For this review, take the finished solid that the model builds, in its own axes (mm). A direction names the side the tool comes from. Give positions to 0.01 mm unless a question says otherwise; leave off trailing zeros. Write each loop counter-clockwise with the first axis right and the second up, starting at its lowest first coordinate (ties: lowest second). Pieces come first, ordered by that corner, then holes. Notation, with made-up numbers: (53.25, 32.5) -> (111.25, 32.5) arc R28 cw to (111.25, 56.5) -> close; hole circle Ø5 at (61, 17.5). An arc over 180 degrees is marked (long way). Return JSON: item names as keys, results as strings.
from build123d import *

# Parameters (mm, degrees)
SKETCH1_R           = 2
SKETCH1_R_2         = 1.025
BOSS_EXTRUDE1_DEPTH = 3
SKETCH2_R           = 2
BOSS_EXTRUDE2_DEPTH = 1
SKETCH3_R           = 1.575
BOSS_EXTRUDE3_DEPTH = 27


with BuildPart() as part:
    # Sketch1 → Boss-Extrude1 (new body)
    with BuildSketch(Plane(origin=(0, 0, 0), x_dir=(1, 0, 0), z_dir=(0, 1, 0))):
        Circle(SKETCH1_R)
        Circle(SKETCH1_R_2, mode=Mode.SUBTRACT)
    extrude(amount=BOSS_EXTRUDE1_DEPTH)

    # Sketch2 → Boss-Extrude2 (add)
    with BuildSketch(Plane(origin=(0, 3, 0), x_dir=(1, 0, 0), z_dir=(0, 1, 0))):
        Circle(SKETCH2_R)
    extrude(amount=BOSS_EXTRUDE2_DEPTH)

    # Sketch3 → Boss-Extrude3 (add)
    with BuildSketch(Plane(origin=(0, 4, 0), x_dir=(1, 0, 0), z_dir=(0, 1, 0))):
        Circle(SKETCH3_R)
    extrude(amount=BOSS_EXTRUDE3_DEPTH)


solid = part.part
1. The part is to be moulded in two halves that separate along Z. For faces 3 (the cylindrical face through (-0.133, 1.479, -1.016)), 4 (the flat face through (0, 31, 0)), 5 (the cylindrical face through (-1.25, 17.31, 0.96)), say which applies: +Z half, -Z half, draft (parallel to the pull), parting line (faces both ways), or undercut.
Results found:
{"face 3": "undercut", "face 4": "draft", "face 5": "parting line"}
2. For pin 1 (1.5 mm diameter, centred on x = -1, z = 0.5, fed in from -Y); pin 2 (1 mm diameter, centred on x = 0, z = 0, fed in from -Y), all flat-tipped, find the tip position at first contact; note any pin that passes through.
Results found:
{"pin 1": "stops at y = 0", "pin 2": "stops at y = 3"}
3. Add section C-C, the plane y = 4.5. State the section outline as (x, z) points (3 decimals), plus the area to 3 significant figures.
Results found:
{"outline": "circle Ø3.15 at (0, 0)", "area": "7.79 mm²"}
4. Add section B-B, the plane x = 0. State the section outline as (y, z) points (3 decimals), plus the area to 3 significant figures.
Results found:
{"outline": "(0, -2) -> (4, -2) -> (4, -1.575) -> (31, -1.575) -> (31, 1.575) -> (4, 1.575) -> (4, 2) -> (0, 2) -> (0, 1.025) -> (3, 1.025) -> (3, -1.025) -> (0, -1.025) -> close", "area": "94.9 mm²"}
5. Add section A-A, the plane z = 0. State the section outline as (x, y) points (3 decimals), plus the area to 3 significant figures.
Results found:
{"outline": "(-2, 0) -> (-1.025, 0) -> (-1.025, 3) -> (1.025, 3) -> (1.025, 0) -> (2, 0) -> (2, 4) -> (1.575, 4) -> (1.575, 31) -> (-1.575, 31) -> (-1.575, 4) -> (-2, 4) -> close", "area": "94.9 mm²"}
6. To check wall thickness, follow probe 1 along X at (y, z) = (1.4, 0) (3 decimals); probe 2 along Y at (x, z) = (-0.65, -0.5). State the ranges of each line that lie inside material, in increasing order.
Results found:
{"probe 1": "x = -2 to -1.025, 1.025 to 2", "probe 2": "y = 3 to 31"}
7. For faces 1 (the flat face through (0, 3, 0)), 2 (the flat face through (1, 0, 1)), list the 3-axis set-ups (+Z, -Z, +X, -X, +Y, -Y) from which the entire face can be reached by the end or side of a thin tool; tool diameter is ignored.
Results found:
{"face 1": "-Y", "face 2": "+Z, -Z, +X, -X, -Y"}
